```python
from build123d import *

# Parameters (mm, degrees)
SKETCH1_R           = 0.9
SKETCH1_W           = 4.2
SKETCH1_H           = 8
SKETCH1_H_2         = 6
BOSS_EXTRUDE1_DEPTH = 2


with BuildPart() as part:
    # Sketch1 → Boss-Extrude1 (new body)
    with BuildSketch(Plane.XY):
        with BuildLine():
            Line((4, 26), (2, 26))
            ThreePointArc((2, 26), (0.585786438, 26.585786438), (0, 28))
            Line((0, 28), (0, 53.14))
            ThreePointArc((0, 53.14), (0.585786438, 54.554213562), (2, 55.14))
            Line((2, 55.14), (4, 55.14))
            Line((4, 55.14), (4, 63.14))
            Line((4, 63.14), (2, 63.14))
            ThreePointArc((2, 63.14), (0.585786438, 63.725786438), (0, 65.14))
            Line((0, 65.14), (0, 84.665))
            ThreePointArc((0, 84.665), (0.585786438, 86.079213562), (2, 86.665))
            Line((2, 86.665), (4, 86.665))
            Line((4, 86.665), (4, 92.665))
            Line((4, 92.665), (2, 92.665))
            ThreePointArc((2, 92.665), (0.585786438, 93.250786438), (0, 94.665))
            Line((0, 94.665), (0, 104.46))
            Line((0, 104.46), (16.2, 104.46))
            Line((16.2, 104.46), (16.2, 94.665))
            ThreePointArc((16.2, 94.665), (15.614213562, 93.250786438), (14.2, 92.665))
            Line((14.2, 92.665), (12.2, 92.665))
            Line((12.2, 92.665), (12.2, 86.665))
            Line((12.2, 86.665), (14.2, 86.665))
            ThreePointArc((14.2, 86.665), (15.614213562, 86.079213562), (16.2, 84.665))
            Line((16.2, 84.665), (16.2, 65.14))
            ThreePointArc((16.2, 65.14), (15.614213562, 63.725786438), (14.2, 63.14))
            Line((14.2, 63.14), (12.2, 63.14))
            Line((12.2, 63.14), (12.2, 55.14))
            Line((12.2, 55.14), (14.2, 55.14))
            ThreePointArc((14.2, 55.14), (15.614213562, 54.554213562), (16.2, 53.14))
            Line((16.2, 53.14), (16.2, 28))
            ThreePointArc((16.2, 28), (15.614213562, 26.585786438), (14.2, 26))
            Line((14.2, 26), (12.2, 26))
            Line((12.2, 26), (12.2, 14))
            Line((12.2, 14), (10.2, 14))
            Line((10.2, 14), (10.2, 26))
            Line((10.2, 26), (6, 26))
            Line((6, 26), (6, 14))
            Line((6, 14), (4, 14))
            Line((4, 14), (4, 26))
        make_face()
        with Locations((13.45, 94.665)):
            Circle(SKETCH1_R, mode=Mode.SUBTRACT)
        with Locations((13.45, 84.165)):
            Circle(SKETCH1_R, mode=Mode.SUBTRACT)
        with Locations((13.45, 65.64)):
            Circle(SKETCH1_R, mode=Mode.SUBTRACT)
        with Locations((13.45, 52.64)):
            Circle(SKETCH1_R, mode=Mode.SUBTRACT)
        with Locations((13.45, 28.5)):
            Circle(SKETCH1_R, mode=Mode.SUBTRACT)
        with Locations((10.2, 35.5)):
            Circle(SKETCH1_R, mode=Mode.SUBTRACT)
        with Locations((10.2, 45.64)):
            Circle(SKETCH1_R, mode=Mode.SUBTRACT)
        with Locations((13.45, 100.665)):
            Circle(SKETCH1_R, mode=Mode.SUBTRACT)
        with Locations((2.75, 100.665)):
            Circle(SKETCH1_R, mode=Mode.SUBTRACT)
        with Locations((6, 45.64)):
            Circle(SKETCH1_R, mode=Mode.SUBTRACT)
        with Locations((6, 35.5)):
            Circle(SKETCH1_R, mode=Mode.SUBTRACT)
        with Locations((2.75, 28.5)):
            Circle(SKETCH1_R, mode=Mode.SUBTRACT)
        with Locations((2.75, 52.64)):
            Circle(SKETCH1_R, mode=Mode.SUBTRACT)
        with Locations((2.75, 65.64)):
            Circle(SKETCH1_R, mode=Mode.SUBTRACT)
        with Locations((2.75, 84.165)):
            Circle(SKETCH1_R, mode=Mode.SUBTRACT)
        with Locations((2.75, 94.665)):
            Circle(SKETCH1_R, mode=Mode.SUBTRACT)
        with Locations((8.1, 59.14)):
            Rectangle(SKETCH1_W, SKETCH1_H, mode=Mode.SUBTRACT)
        with Locations((8.1, 89.665)):
            Rectangle(SKETCH1_W, SKETCH1_H_2, mode=Mode.SUBTRACT)
    extrude(amount=BOSS_EXTRUDE1_DEPTH)


solid = part.part
```
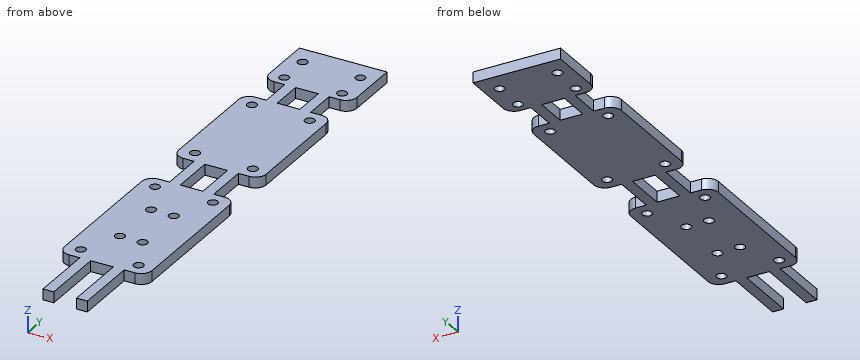
Could you check a few things on this model? Use its own coordinates, in mm. Give positions to 0.01 mm unless a question says otherwise; leave off trailing zeros. Order: outer loops, then holes, each group sorted by start corner. A loop starts at its lowest first (then second) coordinate and runs counter-clockwise, first axis right, second up.
Q1. I'm going to push flat-ended pins straight in: P1, Ø1, axis at y = 61, z = 0.5, coming from the -X side; P2, Ø2.5, axis at x = 2.75, y = 28.5, coming from the +Z side; P3, Ø0.6, axis at x = 7.5, z = 1, coming from the -Y side. Where does each tip first touch, or does it pass through?
Q2. If I drill on line 1 along X through (y, z) = (52.64, 1.15); line 2 along X through (y, z) = (35.5, 0.65); line 3 along Y through (x, z) = (8.5, 1.7) (3 decimals), over which ranges is the centre line in solid material (lowest first)?
Q3. Suppose I cut it at A-A, the plane y = 45.64. Write out the boundary of the cut face in (x, z), and give its area (3 significant figures).
Q4. Suppose I cut it at B-B, the plane x = 13.45. Count the separate pieces of the cut face and the enclosed holes in it, and give its area (3 significant figures).
Solution:
1. P1: stops at x = 4
1. P2: stops at z = 2
1. P3: stops at y = 26
2. line 1: x = 0 to 1.85, 3.65 to 12.55, 14.35 to 16.2
2. line 2: x = 0 to 5.1, 6.9 to 9.3, 11.1 to 16.2
2. line 3: y = 26 to 55.14, 63.14 to 86.665, 92.665 to 104.46
3. outline: (0, 0) - (5.1, 0) - (5.1, 2) - (0, 2) - close; (6.9, 0) - (9.3, 0) - (9.3, 2) - (6.9, 2) - close; (11.1, 0) - (16.2, 0) - (16.2, 2) - (11.1, 2) - close
3. area: 25.2 mm2
4. separate pieces: 9
4. enclosed holes: 0
4. area: 107 mm2
